Input: part model. Units: mm. Frame: model coordinates. A direction names the side the tool comes from. Give positions to 0.01 mm unless a question says otherwise; leave off trailing zeros. Loops run counter-clockwise (first coordinate to the right, second up) from the corner with the lowest first, then second, coordinate; pieces in that order, holes last. Notation, with made-up numbers: (5.25, -26) - (26.25, -26) arc R14 cw to (26.25, -20) - close; hole circle Ø9 at (66, -23). An arc over 180 degrees is marked (long way). One line per item, written item: value.
from build123d import *

# Parameters (mm, degrees)
F0_W          = 38.1
F0_H          = 38.1
F1_DEPTH      = 739.775
F3_DEPTH      = 25.4
F6_DEPTH      = 169.8625
F6_DEPTH_BACK = 169.8625


with BuildPart() as f1:
    # F0 (on Top) → F1 (new body)
    with BuildSketch(Plane.XY):
        with Locations((-150.8125, 150.8125)):
            Rectangle(F0_W, F0_H)
        with Locations((-150.8125, -150.8125)):
            Rectangle(F0_W, F0_H)
        with Locations((150.8125, -150.8125)):
            Rectangle(F0_W, F0_H)
        with Locations((150.8125, 150.8125)):
            Rectangle(F0_W, F0_H)
    extrude(amount=F1_DEPTH)


with BuildPart() as f3:
    # F2 (on face) → F3 (new body)
    with BuildSketch(Plane.XY.offset(739.775)):
        Polygon((169.8625, 169.8625), (-131.7625, 169.8625), (-131.7625, 131.7625), (-169.8625, 131.7625), (-169.8625, -169.8625), (169.8625, -169.8625), align=None)
    extrude(amount=-F3_DEPTH)

    # F4: union F1
    add(f1.part)

    # F5 (on Right) → F6 (join, two sides)
    with BuildSketch(Plane.YZ) as f6_sk:
        Polygon((-169.8625, 739.775), (-160.192227, 739.775), (-211.1375, 1028.7), (-236.151617, 1024.289336), (-169.8625, 648.345073), align=None)
    extrude(amount=F6_DEPTH)
    extrude(f6_sk.sketch, amount=-F6_DEPTH_BACK)


solid = f3.part
Item 1: Material intervals for L1, parallel to X at y = -135, z = 458; L2, parallel to Z at x = 136, y = 17 (3 decimals), sorted ascending.
Verdict:
L1: x = -169.86 to -131.76, 131.76 to 169.86
L2: z = 714.375 to 739.775
Item 2: Section B-B, the plane x = -93.5. Output: boundary loops of the cut face in (y, z) (1 decimal).
Verdict:
outline: (-236.2, 1024.3) - (-169.9, 648.3) - (-169.9, 714.4) - (169.9, 714.4) - (169.9, 739.8) - (-160.2, 739.8) - (-211.1, 1028.7) - close
Item 3: Pin query (flat end, axial travel): P1, Ø3, axis at x = -56, y = 114.5, coming from the +Z side (3 decimals); P2, Ø5, axis at x = 33.5, z = 661.5, coming from the +Y side; P3, Ø11.5, axis at x = 156, z = 240.5, coming from the -Y side. Return the tip coordinate at first contact, or that it passes through.
Verdict:
P1: stops at z = 739.775
P2: stops at y = -169.86
P3: stops at y = -169.86
Item 4: Section A-A, the plane z = 319. Output: boundary loops of the cut face in (x, y).
Verdict:
outline: (-169.86, -169.86) - (-131.76, -169.86) - (-131.76, -131.76) - (-169.86, -131.76) - close; (-169.86, 131.76) - (-131.76, 131.76) - (-131.76, 169.86) - (-169.86, 169.86) - close; (131.76, -169.86) - (169.86, -169.86) - (169.86, -131.76) - (131.76, -131.76) - close; (131.76, 131.76) - (169.86, 131.76) - (169.86, 169.86) - (131.76, 169.86) - close
Item 5: Access query for faces 1 (the face through (-151, -131.762, 352)), 2 (the face through (2, -169.862, 681)), 3 (the face through (-2, 7, 739.775)), 4 (the face through (151, -169.862, 329)). Directions: +Z, -Z, +X, -X, +Y, -Y. A direction counts if a zero-diameter tool reaches every point of the face in a straight line with its end or side. Return the directions, or none.
Verdict:
face 1: -Z, +X, -X
face 2: -Z, +Y
face 3: +Z, +X, -X, +Y
face 4: -Z, +X, -X, -Y
Item 6: Section C-C, the plane y = 78. Output: boundary loops of the cut face in (x, z) (1 decimal), and give its area (3 significant figures).
Verdict:
outline: (-169.9, 714.4) - (169.9, 714.4) - (169.9, 739.8) - (-169.9, 739.8) - close
area: 8,630 mm^2
Item 7: Section D-D, the plane z = 730.5. Output: boundary loops of the cut face in (x, y), and give its area (3 significant figures).
Verdict:
outline: (-169.86, -184.35) - (169.86, -184.35) - (169.86, 169.86) - (-169.86, 169.86) - close
area: 120,000 mm^2
Item 8: Draft query along Y for faces 5 (the face through (-139, 169.862, 423)), 6 (the face through (131.762, -151, 352)), 7 (the face through (151, 131.762, 352)). Return one class per face: pulls with the +Y half, pulls with the -Y half, needs draft (parallel to the pull), parting line crosses it, or undercut.
Verdict:
face 5: pulls with the +Y half
face 6: needs draft
face 7: undercut
